Autodesk Inventor part; units mm, degrees
ref_plane "YZ Plane" through (0, 0, 0) normal (1, 0, 0) x (0, 1, 0)
ref_plane "XZ Plane" through (0, 0, 0) normal (0, 1, 0) x (-1, 0, 0)
ref_plane "XY Plane" through (0, 0, 0) normal (0, 0, 1) x (1, 0, 0)
sketch "Sketch1" plane through (0, 0, 0) normal (0, 0, 1) x (1, 0, 0)
  line L0 (-490, 81) -> (490, 81)
  line L1 (490, 81) -> (490, 0)
  line L2 (490, 0) -> (-490, 0)
  line L3 (-490, 0) -> (-490, 81)
  point P0 (0, 0)
  point P1 (0, 0)
  dimension "d0" = 980
  dimension "d1" = 81
extrude "Plate1" add sketch "Sketch1" along normal blind 2
sketch "Sketch2" plane through (490, -2, 0) normal (0, 1, 0) x (-1, 0, 0)
  line L0 (980, 0) -> (0, 0)
  line L1 (0, 0) -> (0, 20)
  line L2 (0, 20) -> (980, 20)
  line L3 (980, 20) -> (980, 0)
edge flange "Flange1" height 20 angle 90 thickness 2 bend radius 2.75 thickness toward (0, 1, 0) relief round relief width 2 relief depth 1 edges at (0, 0, 2) wall of the first edge with corners at (-490, -2, 0) (490, -2, 0) (490, -2, 20) (-490, -2, 20)
bend "Bend1"
corner "Corner1"
sketch "Sketch5" plane through (0, 0, 0) normal (0, 0, -1) x (-1, 0, 0)
  line L0 (490, 81) -> (-490, 81)
  line L1 (490, -2) -> (-490, -2)
  circle A0 centre (0, 81) radius 25
  line L2 (243.95, 81) -> (246.05, 81)
  line L3 (246.05, 81) -> (246.05, 26)
  line L4 (246.05, 26) -> (243.95, 26)
  line L5 (243.95, 26) -> (243.95, 81)
  line L6 (-243.95, 81) -> (-246.05, 81)
  line L7 (-246.05, 81) -> (-246.05, 26)
  line L8 (-246.05, 26) -> (-243.95, 26)
  line L9 (-243.95, 26) -> (-243.95, 81)
  line L10 (0, 81) -> (0, -2) construction
  line L11 (-490, -2) -> (-490, 81)
  line L12 (490, -2) -> (490, 81)
  circle A1 centre (-490, 81) radius 25
  circle A2 centre (490, 81) radius 25
  point P0 (0, 0)
  point P1 (245, 26)
  point P2 (-245, 26)
  point P3 (246.05, 81)
  point P4 (-25, 81)
  point P5 (25, 81)
  point P6 (-246.05, 81)
  point P7 (465, 81)
  point P8 (490, 56)
  point P9 (-490, 56)
  point P10 (-465, 81)
  dimension "d45" = 50
  dimension "d48" = 2.1
  dimension "d49" = 490
  dimension "d51" = 28
  dimension "d52" = 55
extrude "Extrusion1" cut sketch "Sketch5" against normal through all contours L3 L4 L5 L0 | L0 L12 A2 | L9 L8 L7 L0 | L11 L0 A1 picked at (488.1457, 64.5423) picked at (-481.1886, 66.9767)
sketch "Sketch9" plane through (0, 0, 2) normal (0, 0, 1) x (1, 0, 0)
  line L0 (467.0539, 27.7998) -> (467.0539, 15.7998) construction
  line L1 (467.0539, 15.7998) -> (267.0539, 15.7998) construction
  line L2 (267.0539, 15.7998) -> (267.0539, 27.7998) construction
  line L3 (267.0539, 27.7998) -> (467.0539, 27.7998) construction
  line L4 (-490, 81) -> (490, 81)
  point P0 (0, 0)
  point P1 (1.05, 68)
  point P2 (490, 81)
  point P3 (-490, 81)
  dimension "d40" = 200
  dimension "d41" = 12
mark "Mark2"
equation "\"d2\" = Thickness"
equation "\"d3\" = BendReliefWidth"
equation "\"d4\" = BendReliefDepth"
equation "\"d5\" = MinimumRemnant"
equation "\"d6\" = TransitionRadius"
equation "\"d9\" = BendRadius"
equation "\"d10\" = CornerReliefSize"
equation "\"d11\" = GapSize"
equation "\"d12\" = JacobiRadiusSize"
equation "\"BendReliefWidth\" = Thickness"
equation "\"BendReliefDepth\" = 0.5 * Thickness"
equation "\"CornerReliefSize\" = 4 * Thickness"
equation "\"MinimumRemnant\" = 2 * Thickness"
equation "\"TransitionRadius\" = BendRadius"
equation "\"JacobiRadiusSize\" = BendRadius"
equation "\"GapSize\" = Thickness"
properties part number "MSC 331 STRINGER BOARD  ####" material "Stainless Steel"
Design review of the part built by this model. Coordinates are the model's own, in mm. A direction names the side the tool comes from. Give positions to 0.01 mm unless a question says otherwise; leave off trailing zeros. Loops run counter-clockwise (first coordinate to the right, second up) from the corner with the lowest first, then second, coordinate; pieces in that order, holes last. Notation, with made-up numbers: (-22, 8) -> (-12, 8) arc R12 ccw to (-12, 25) -> close; hole circle Ø11 at (69.25, 67). An arc over 180 degrees is marked (long way). One line per item, written item: value.
Q1. We need section A-A on y = 46. Give the boundary of the cut face in (x, z).
Numbers:
outline: (-490, 0) -> (-246.05, 0) -> (-246.05, 2) -> (-490, 2) -> close; (-243.95, 0) -> (243.95, 0) -> (243.95, 2) -> (-243.95, 2) -> close; (246.05, 0) -> (490, 0) -> (490, 2) -> (246.05, 2) -> close
Q2. For L1, parallel to X at y = 47.5, z = 1.75; L2, parallel to X at y = 73, z = 1.5; L3, parallel to Y at x = -10.5, z = 16, list the stretches that pass through material, from the lowest coordinate up.
Numbers:
L1: x = -490 to -246.05, -243.95 to 243.95, 246.05 to 490
L2: x = -466.31 to -246.05, -243.95 to 243.95, 246.05 to 466.31
L3: y = -2 to 0
Q3. For pin 1 Ø1.6 at (y, z) = (66.5, 1) entering from -X; pin 2 Ø2 at (x, y) = (280.5, 34.5) entering from +Z; pin 3 Ø7.5 at (x, z) = (-30, 9) entering from +Y, all flat-tipped, find the tip position at first contact; note any pin that passes through.
Numbers:
pin 1: stops at x = -470.23
pin 2: stops at z = 2
pin 3: stops at y = 0
Q4. We need section C-C on z = 8.5. Give the boundary of the cut face in (x, y), and give its area (3 significant figures).
Numbers:
outline: (-490, -2) -> (490, -2) -> (490, 0) -> (-490, 0) -> close
area: 1,960 mm^2
Q5. We need section B-B on x = -323. Give the boundary of the cut face in (y, z), and give its area (3 significant figures).
Numbers:
outline: (-2, 4.75) arc R4.75 ccw to (2.75, 0) -> (81, 0) -> (81, 2) -> (2.75, 2) arc R2.75 cw to (0, 4.75) -> (0, 20) -> (-2, 20) -> close
area: 199 mm^2
Q6. Machinability: for faces 1 (the flat face through (490, 20, 1)), 2 (the flat face through (-7, 42, 2)), which of the approach directions +Z, -Z, +X, -X, +Y, -Y give a long, thin tool a straight path to every point of the face, cutting with its end or side? Answer none if there is none.
Numbers:
face 1: +Z, -Z, +X, +Y, -Y
face 2: +Z, +X, -X, +Y
